Verification items for this drawing (mm, ordinates from the low corner). Give positions to 0.01 mm unless a question says otherwise; leave off trailing zeros. Loops run counter-clockwise (first coordinate to the right, second up) from the corner with the lowest first, then second, coordinate; pieces in that order, holes last. Notation, with made-up numbers: M 87,3 L 146,3 A15 ccw 146,15 Z; hole C -3.5,-17 d8. An arc over 180 degrees is marked long. Answer in a Markdown table with one row per item.
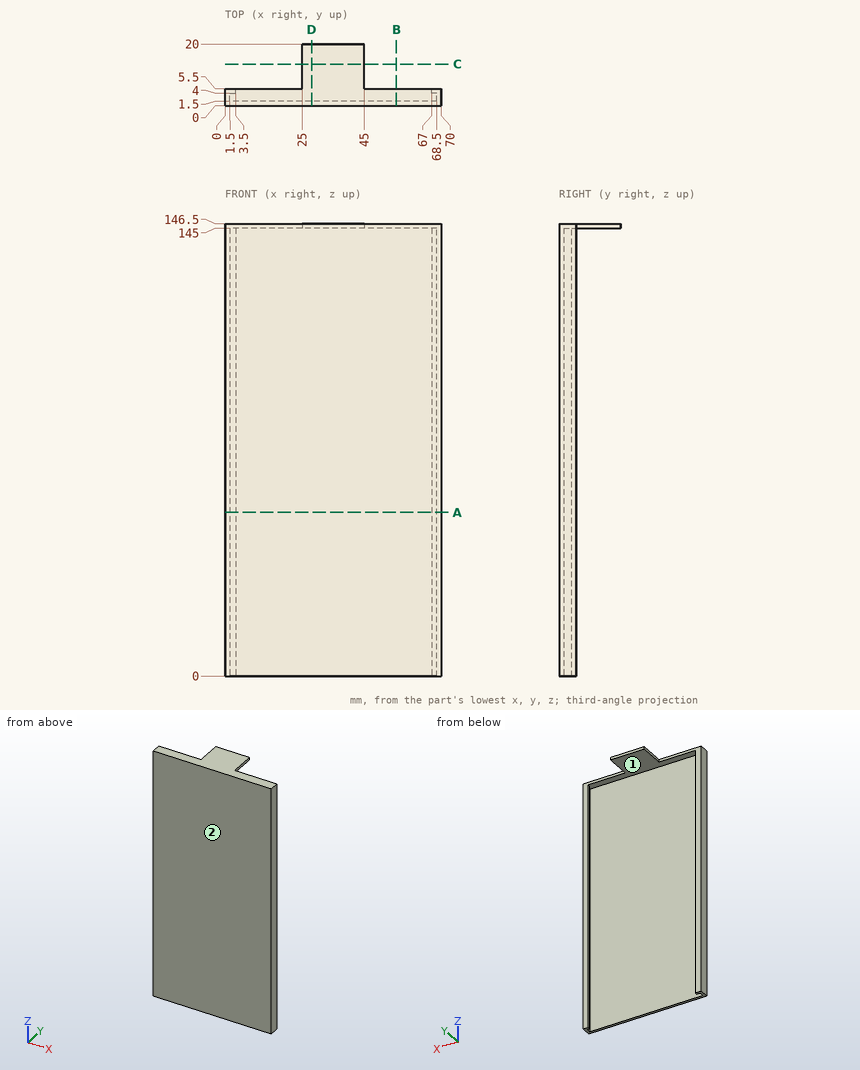
Item 1: Sectioned sample at D-D (x = 28). Record the cut outline in (y, z), and give its area (4 significant figures).
Reported:
| item | result |
|---|---|
| outline | M 0,0 L 1.5,0 L 1.5,145 L 20,145 L 20,146.5 L 0,146.5 Z |
| area | 247.5 mm^2 |
Item 2: Release check for a two-part mould opening along X. For the marked faces 1 and 2 record: released by +X, released by -X, zero draft, split by the parting line, or undercut.
Reported:
| item | result |
|---|---|
| face 1 | undercut |
| face 2 | zero draft |
Item 3: Go/stop test with flat-tipped pins: pin 1 (0.8 mm diameter, centred on x = 67.5, z = 77, fed in from -Y); pin 2 (2 mm diameter, centred on x = 32, z = 116.5, fed in from +Y); pin 3 (1.2 mm diameter, centred on y = 13.5, z = 145.5, fed in from +X); pin 4 (9 mm diameter, centred on x = 21.5, y = 13.5, fed in from -Z). Record where each tip stops, or that it passes through.
Reported:
| item | result |
|---|---|
| pin 1 | stops at y = 0 |
| pin 2 | stops at y = 1.5 |
| pin 3 | stops at x = 45 |
| pin 4 | stops at z = 145 |
Item 4: Sectioned sample at A-A (z = 53). Record the cut outline in (x, y).
Reported:
| item | result |
|---|---|
| outline | M 0,0 L 70,0 L 70,5.5 L 67,5.5 L 67,4 L 68.5,4 L 68.5,1.5 L 1.5,1.5 L 1.5,4 L 3.5,4 L 3.5,5.5 L 0,5.5 Z |
Item 5: Scan lines: L1, parallel to X at y = 4.25, z = 17.5; L2, parallel to Y at x = 31.5, z = 36; L3, parallel to X at y = 2.25, z = 65.5. Record each from-to range of solid material in increasing order. Write a range as [from, to].
Reported:
| item | result |
|---|---|
| L1 | x = [0, 3.5], [67, 70] |
| L2 | y = [0, 1.5] |
| L3 | x = [0, 1.5], [68.5, 70] |
Item 6: Sectioned sample at B-B (x = 55.5). Record the cut outline in (y, z).
Reported:
| item | result |
|---|---|
| outline | M 0,0 L 1.5,0 L 1.5,145 L 5.5,145 L 5.5,146.5 L 0,146.5 Z |
Item 7: Sectioned sample at C-C (y = 13.5). Record the cut outline in (x, z).
Reported:
| item | result |
|---|---|
| outline | M 25,145 L 45,145 L 45,146.5 L 25,146.5 Z |
